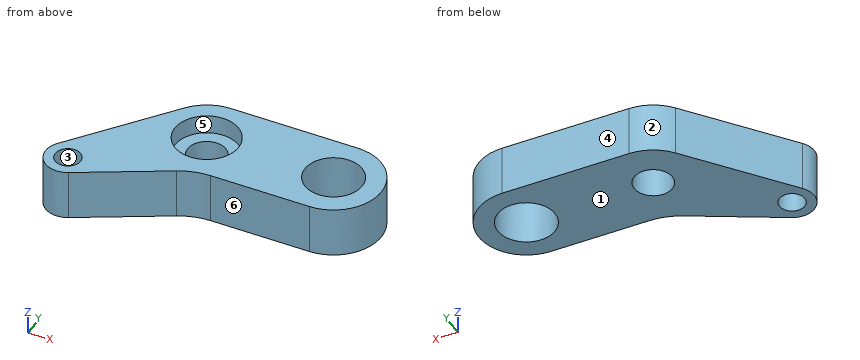
```python
from build123d import *

# Parameters (mm, degrees)
SKETCH_1_R          = 3.5
SKETCH_1_R_2        = 2
SKETCH_1_R_3        = 7.5
SKETCH_1_R_4        = 3
SKETCH_1_R_5        = 4.5
EXTRUDE_1_DEPTH     = 8
FILLET_1_R          = 10
SKETCH_2_R          = 5
CUT_EXTRUDE_1_DEPTH = 3


with BuildPart() as part:
    # Эскиз1 → Бобышка-Вытянуть1 (new body)
    # profile 1 of 6: a face of its own
    with BuildSketch(Plane.XY):
        with Locations((-35.320888862, -12.855752194)):
            Circle(SKETCH_1_R)
        with Locations((-35.320888862, -12.855752194)):
            Circle(SKETCH_1_R_2, mode=Mode.SUBTRACT)
    # profile 2 of 6: a face of its own
    with BuildSketch(Plane.XY):
        with BuildLine():
            ThreePointArc((-20, -7.5), (-26.754185537, -3.260518017), (-25.872571635, 4.665072603))
            Line((-25.872571635, 4.665072603), (-38.061422292, -10.678718312))
            ThreePointArc((-38.061422292, -10.678718312), (-34.168037398, -9.551068623), (-31.820888862, -12.855752194))
            ThreePointArc((-31.820888862, -12.855752194), (-32.313543751, -14.646248042), (-33.652817653, -15.932688729))
            Line((-33.652817653, -15.932688729), (-18.097817426, -7.5))
            Line((-18.097817426, -7.5), (-20, -7.5))
        make_face()
    # profile 3 of 6: a face of its own
    with BuildSketch(Plane.XY):
        with Locations((-20, 0)):
            Circle(SKETCH_1_R_3)
        with Locations((-20, 0)):
            Circle(SKETCH_1_R_4, mode=Mode.SUBTRACT)
    # profile 4 of 6: a face of its own
    with BuildSketch(Plane.XY):
        with BuildLine():
            Line((-20, -7.5), (-18.097817426, -7.5))
            Line((-18.097817426, -7.5), (-16.425561695, -6.593435432))
            ThreePointArc((-16.425561695, -6.593435432), (-18.156194932, -7.26982688), (-20, -7.5))
        make_face()
    # profile 5 of 6: a face of its own
    with BuildSketch(Plane.XY):
        with BuildLine():
            ThreePointArc((0, -7.5), (-7.5, 0), (0, 7.5))
            Line((0, 7.5), (-20, 7.5))
            ThreePointArc((-20, 7.5), (-14.696699141, 5.303300859), (-12.5, 0))
            ThreePointArc((-12.5, 0), (-13.555689048, -3.836776818), (-16.425561695, -6.593435432))
            Line((-16.425561695, -6.593435432), (-18.097817426, -7.5))
            Line((-18.097817426, -7.5), (0, -7.5))
        make_face()
    # profile 6 of 6: a face of its own
    with BuildSketch(Plane.XY):
        Circle(SKETCH_1_R_3)
        Circle(SKETCH_1_R_5, mode=Mode.SUBTRACT)
    extrude(amount=EXTRUDE_1_DEPTH)

    # Скругление1
    fillet_1_edges = [part.edges().sort_by_distance(p)[0] for p in [
        (-18.097817426, -7.5, 4),
    ]]
    fillet(fillet_1_edges, radius=FILLET_1_R)

    # Эскиз2 → Вырез-Вытянуть1 (cut)
    with BuildSketch(Plane.XY.offset(8)):
        with Locations((-20, 0)):
            Circle(SKETCH_2_R)
    extrude(amount=-CUT_EXTRUDE_1_DEPTH, mode=Mode.SUBTRACT)


solid = part.part
```
The listing builds one solid part. Answer for the finished solid, in the listing's coordinates (mm). Face numbers are marked on the shaded views. A direction names the side the tool comes from. Coordinates: 2 decimals unless noted, no trailing zeros. Loops run counter-clockwise (first coordinate to the right, second up) from the corner with the lowest first, then second, coordinate; pieces in that order, holes last. Notation, with made-up numbers: (2.5, 89.5) - (7.5, 89.5) arc R30 ccw to (7.5, 125.5) - close; hole circle Ø3 at (62, 26). An arc over 180 degrees is marked (long way). Use a Markdown table: item, result. Add a question column.
1) For the marked faces 4, 5 and 6, determine the directions among +Z, -Z, +X, -X, +Y, -Y from which every point of the face is accessible in a straight line to the end or side of a thin tool.
2) The mould has two halves that part along X. Classify the marked faces 1, 2 and 3: released by +X, released by -X, zero draft, split by the parting line, or undercut.
3) Given pin 1 (8 mm diameter, centred on x = -20, y = 0, fed in from +Z); pin 2 (2.5 mm diameter, centred on x = -8.5, z = 6, fed in from -Y); pin 3 (5.5 mm diameter, centred on x = -20, y = 0, fed in from -Z); pin 4 (3 mm diameter, centred on y = 2, z = 6, fed in from +X), each flat-ended and moving along its own axis, determine where each tip first touches the part or whether it passes through.
4) The part is cut by section B-B, the plane x = -1. Give the vertices of the cut face in (y, z).
5) The part is cut by section D-D, the plane y = 0. Give the vertices of the cut face in (x, z).
6) Find the intervals of material crossed by line 1 (Y direction, x = 0, z = 4.75); line 2 (X direction, y = -2, z = 1.75); line 3 (X direction, y = -2.25, z = 5.5), in increasing order.
7) The part is cut by section C-C, the plane z = 7. Give the vertices of the cut face in (x, y), and give its area (3 significant figures).
8) The part is cut by section A-A, the plane y = 3.75. Give the vertices of the cut face in (x, z), and give its area (3 significant figures).
Here are the results:
| question | item | result |
|---|---|---|
| 1 | face 4 | +Z, -Z, +X, -X, +Y |
| 1 | face 5 | +Z |
| 1 | face 6 | +Z, -Z, +X, -Y |
| 2 | face 1 | zero draft |
| 2 | face 2 | released by -X |
| 2 | face 3 | undercut |
| 3 | pin 1 | stops at z = 5 |
| 3 | pin 2 | stops at y = -7.5 |
| 3 | pin 3 | passes through |
| 3 | pin 4 | stops at x = 7.48 |
| 4 | outline | (-7.5, 0) - (-4.39, 0) - (-4.39, 8) - (-7.5, 8) - close; (4.39, 0) - (7.5, 0) - (7.5, 8) - (4.39, 8) - close |
| 5 | outline | (-29.58, 0) - (-23, 0) - (-23, 5) - (-25, 5) - (-25, 8) - (-29.58, 8) - close; (-17, 0) - (-4.5, 0) - (-4.5, 8) - (-15, 8) - (-15, 5) - (-17, 5) - close; (4.5, 0) - (7.5, 0) - (7.5, 8) - (4.5, 8) - close |
| 6 | line 1 | y = -7.5 to -4.5, 4.5 to 7.5 |
| 6 | line 2 | x = -31.17 to -22.24, -17.76 to -4.03, 4.03 to 7.23 |
| 6 | line 3 | x = -31.37 to -24.47, -15.53 to -3.9, 3.9 to 7.15 |
| 7 | outline | (-38.06, -10.68) arc R3.5 ccw to (-33.65, -15.93) - (-20.33, -8.71) arc R10 cw to (-15.56, -7.5) - (0, -7.5) arc R7.5 ccw to (0, 7.5) - (-20, 7.5) arc R7.5 ccw to (-25.87, 4.67) - close; hole circle Ø4 at (-35.32, -12.86); hole circle Ø10 at (-20, 0); hole circle Ø9 at (0, 0) |
| 7 | area | 478 mm^2 |
| 8 | outline | (-26.6, 0) - (-2.49, 0) - (-2.49, 8) - (-16.69, 8) - (-16.69, 5) - (-23.31, 5) - (-23.31, 8) - (-26.6, 8) - close; (2.49, 0) - (6.5, 0) - (6.5, 8) - (2.49, 8) - close |
| 8 | area | 205 mm^2 |
